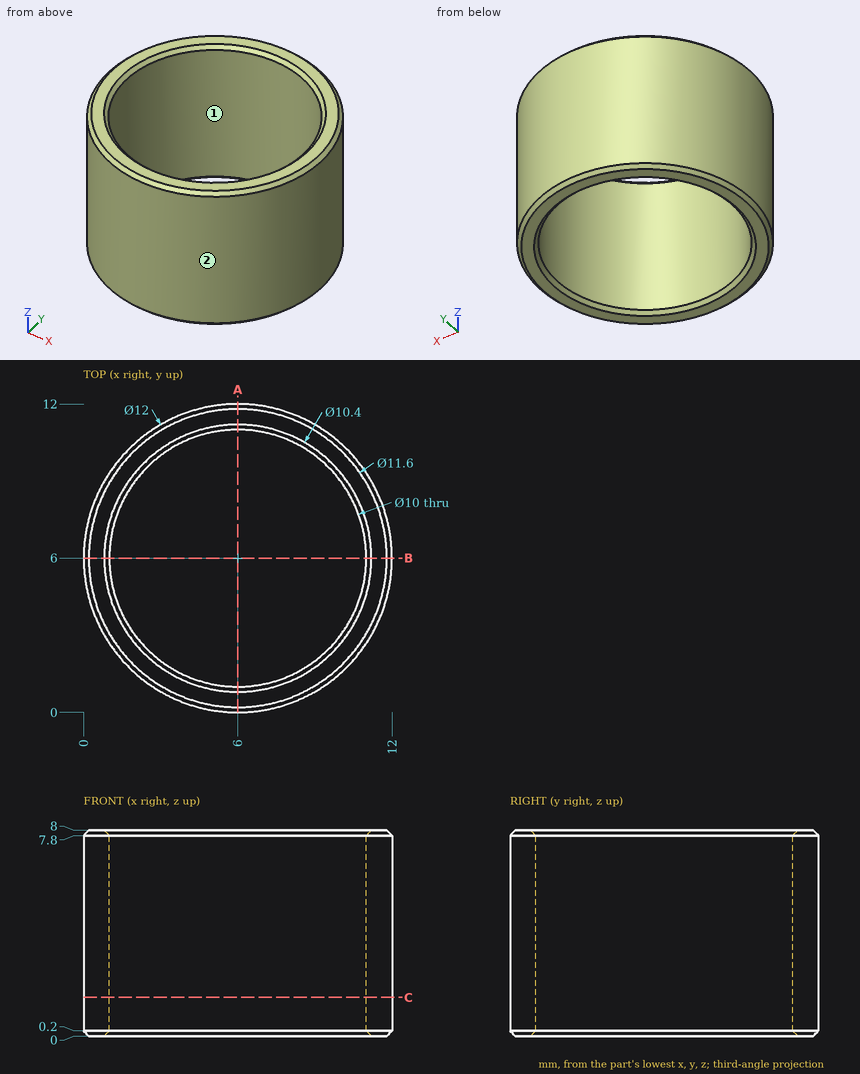
Here's the drawing with two shaded views (mm, measured from the low corner). I have some questions. Coordinates: 2 decimals unless noted, no trailing zeros. Order: outer loops, then holes, each group sorted by start corner. A loop starts at its lowest first (then second) coordinate and runs counter-clockwise, first axis right, second up.
Q1. Thinking about a two-plate mould opening in X: for the marked faces 1 and 2, which applies, released by +X, released by -X, zero draft, split by the parting line, or undercut?
Q2. Please list where these lines run through material, in increasing order: L1, parallel to Y at x = 6, z = 6; L2, parallel to X at y = 5.75, z = 5.5; L3, parallel to X at y = 4.25, z = 4.75.
Q3. Suppose I cut it at A-A on x = 6. Please give me the cut outline in (y, z), and give its area (3 significant figures).
Q4. Suppose I cut it at C-C on z = 1.5. Please give me the cut outline in (x, y), and give its area (3 significant figures).
Q5. Will these pins go through, and if not, where does the flat tip stop? pin 1 (1.5 mm diameter, centred on y = 4.5, z = 1.5, fed in from -X); pin 2 (1.5 mm diameter, centred on x = 9, y = 6, fed in from -Z); pin 3 (2 mm diameter, centred on y = 4, z = 6.5, fed in from -X).
Answer:
1. face 1: undercut
1. face 2: split by the parting line
2. L1: y = 0 to 1, 11 to 12
2. L2: x = 0.01 to 1.01, 10.99 to 11.99
2. L3: x = 0.26 to 1.32, 10.68 to 11.74
3. outline: (0, 0.2) - (0.2, 0) - (0.8, 0) - (1, 0.2) - (1, 7.8) - (0.8, 8) - (0.2, 8) - (0, 7.8) - close; (11, 0.2) - (11.2, 0) - (11.8, 0) - (12, 0.2) - (12, 7.8) - (11.8, 8) - (11.2, 8) - (11, 7.8) - close
3. area: 15.8 mm2
4. outline: circle Ø12 at (6, 6); hole circle Ø10 at (6, 6)
4. area: 34.6 mm2
5. pin 1: stops at x = 0.05
5. pin 2: passes through
5. pin 3: stops at x = 0.08
